Check sheet for the modelled part. Datum: model origin and axes. Units: mm. Give positions to 0.01 mm unless a question says otherwise; leave off trailing zeros. Loops run counter-clockwise (first coordinate to the right, second up) from the corner with the lowest first, then second, coordinate; pieces in that order, holes last. Notation, with made-up numbers: (-21, -25) - (6, -25) arc R3 ccw to (6, -21) - close; hole circle Ø7 at (63.25, 74.5). An arc over 180 degrees is marked (long way). Use CSV: the item, a comma, the result in double quotes.
Autodesk Inventor part; units mm, degrees
ref_plane "YZ Plane" through (0, 0, 0) normal (1, 0, 0) x (0, 1, 0)
ref_plane "XZ Plane" through (0, 0, 0) normal (0, 1, 0) x (-1, 0, 0)
ref_plane "XY Plane" through (0, 0, 0) normal (0, 0, 1) x (1, 0, 0)
sketch "Sketch1" plane through (0, 0, 0) normal (0, 0, 1) x (1, 0, 0)
  circle A0 centre (0, 0) radius 12.5
  circle A1 centre (0, 0) radius 21
  line L0 (0, 0) -> (-28, 0)
  line L1 (0, 0) -> (28, 0)
  circle A2 centre (-28, 0) radius 1
  circle A3 centre (28, 0) radius 1
  line L2 (0, 0) -> (-35, 0)
  line L3 (0, 0) -> (35, 0)
  line L4 (-35, -4) -> (-35, 4)
  line L5 (35, 4) -> (35, -4)
  line L6 (-35, 4) -> (-10.5231, 18.1732)
  line L7 (-35, -4) -> (-10.5231, -18.1732)
  line L8 (35, 4) -> (10.5231, 18.1732)
  line L9 (35, -4) -> (10.5231, -18.1732)
  dimension "d0" = 25
  dimension "d1" = 42
  dimension "d2" = 28
  dimension "d3" = 28
  dimension "d4" = 2
  dimension "d5" = 2
  dimension "d6" = 35
  dimension "d7" = 35
  dimension "d8" = 8
  dimension "d9" = 4
  dimension "d10" = 8
  dimension "d11" = 4
extrude "Extrusion1" add sketch "Sketch1" along normal blind 7 contours L1 A3 L3 L5 L9 A1 | A1 L8 L5 L3 A3 L1 | L0 A2 L2 L4 L6 A1 | A1 L7 L4 L2 A2 L0
sketch "Sketch2" plane through (0, 0, 0) normal (0, 0, -1) x (-1, 0, 0)
  circle A0 centre (0, 0) radius 21
  circle A1 centre (0, 0) radius 12.5
  dimension "d14" = 25
extrude "Extrusion2" add sketch "Sketch2" against normal blind 11
equation "\"d9\" = 0.5 * d8"
equation "\"d11\" = 0.5 * d10"
properties part number "PneumaticHolder"
1. Sectioned sample at A-A, the plane y = 0. Record the boundary of the cut face in (x, z), and give its area (3 significant figures).
Completed:
outline,"(-35, 0) - (-29, 0) - (-29, 7) - (-35, 7) - close; (-27, 0) - (-12.5, 0) - (-12.5, 11) - (-21, 11) - (-21, 7) - (-27, 7) - close; (12.5, 0) - (27, 0) - (27, 7) - (21, 7) - (21, 11) - (12.5, 11) - close; (29, 0) - (35, 0) - (35, 7) - (29, 7) - close"
area,"355 mm²"
2. Sectioned sample at D-D, the plane y = -10. Record the boundary of the cut face in (x, z).
Completed:
outline,"(-24.64, 0) - (-7.5, 0) - (-7.5, 11) - (-18.47, 11) - (-18.47, 7) - (-24.64, 7) - close; (7.5, 0) - (24.64, 0) - (24.64, 7) - (18.47, 7) - (18.47, 11) - (7.5, 11) - close"
3. Go/stop test with flat-tipped pins: pin 1 Ø1.8 at (x, y) = (28, 0) entering from +Z; pin 2 Ø6 at (x, z) = (-25.5, 7.5) entering from +Y; pin 3 Ø2 at (x, z) = (-6, 9) entering from -Y; pin 4 Ø2 at (x, z) = (-13, 2.5) entering from -Y. Record where each tip stops, or that it passes through.
Completed:
pin 1,"passes through"
pin 2,"stops at y = 11.21"
pin 3,"stops at y = -20.4"
pin 4,"stops at y = -17.32"
4. Sectioned sample at C-C, the plane z = 1.25. Record the boundary of the cut face in (x, y), and give its area (3 significant figures).
Completed:
outline,"(-35, -4) - (-10.52, -18.17) arc R21 ccw to (10.52, -18.17) - (35, -4) - (35, 4) - (10.52, 18.17) arc R21 ccw to (-10.52, 18.17) - (-35, 4) - close; hole circle Ø2 at (-28, 0); hole circle Ø25 at (0, 0); hole circle Ø2 at (28, 0)"
area,"1,430 mm²"
5. Release check for a two-part mould opening along X. For faces 1 (the face through (4.55, -20.5, 6.65)), 2 (the face through (-29, 0, 3)), 3 (the face through (8, 10, 0)) record: released by +X, released by -X, zero draft, split by the parting line, or undercut.
Completed:
face 1,"split by the parting line"
face 2,"undercut"
face 3,"zero draft"
6. Scan lines: line 1 along Y through (x, z) = (0, 3); line 2 along Y through (x, z) = (28, 1.5); line 3 along X through (y, z) = (10.5, 3.5). Record each from-to range of solid material in increasing order.
Completed:
line 1,"y = -21 to -12.5, 12.5 to 21"
line 2,"y = -8.05 to -1, 1 to 8.05"
line 3,"x = -23.77 to -6.78, 6.78 to 23.77"
7. Sectioned sample at B-B, the plane x = 28. Record the boundary of the cut face in (y, z), and give its area (3 significant figures).
Completed:
outline,"(-8.05, 0) - (-1, 0) - (-1, 7) - (-8.05, 7) - close; (1, 0) - (8.05, 0) - (8.05, 7) - (1, 7) - close"
area,"98.7 mm²"
